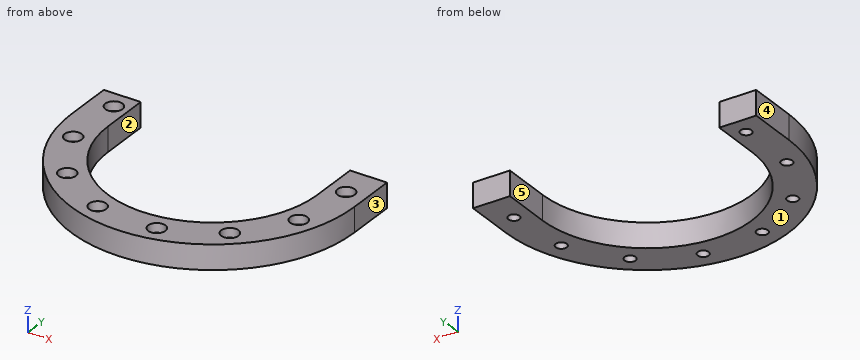
Autodesk Inventor part; units mm, degrees
ref_plane "YZ Plane" through (0, 0, 0) normal (1, 0, 0) x (0, 1, 0)
ref_plane "XZ Plane" through (0, 0, 0) normal (0, 1, 0) x (-1, 0, 0)
ref_plane "XY Plane" through (0, 0, 0) normal (0, 0, 1) x (1, 0, 0)
sketch "Sketch1" plane through (0, 0, 0) normal (0, 0, 1) x (1, 0, 0)
  circle A0 centre (0, 0) radius 200 construction
  line L0 (0, 200) -> (0, 230) construction
  line L1 (0, 200) -> (0, 170) construction
  circle A1 centre (0, 0) radius 170
  circle A2 centre (0, 0) radius 230
  line L2 (-170, 0) -> (-170, 80)
  line L3 (-170, 80) -> (-230, 80)
  line L4 (-230, 80) -> (-230, 0)
  line L5 (170, 0) -> (170, 80)
  line L6 (170, 80) -> (230, 80)
  line L7 (230, 80) -> (230, 0)
  dimension "d13" = 400
  dimension "d26" = 80
  dimension "d36" = 60
extrude "Extrusion1" add sketch "Sketch1" against normal blind 40 contours L5 L6 A2 L3 L2 A1 | L6 L7 A2 | A2 L4 L3 picked at (-188.7937, 40.2131)
sketch "Sketch4" plane through (0, 0, 0) normal (0, 0, 1) x (1, 0, 0)
  circle A0 centre (39.0181, -196.1571) radius 9
  line L0 (0, 0) -> (39.0181, -196.1571) construction
  line L1 (0, 0) -> (0, -276.8337) construction
  dimension "d17" = 18
  dimension "d27" = 200
  dimension "d35" = 11.25
extrude "Extrusion4" cut sketch "Sketch4" against normal through all
sketch "Sketch5" plane through (0, 0, 0) normal (0, 0, 1) x (1, 0, 0)
  circle A0 centre (39.0181, -196.1571) radius 9
  circle A1 centre (39.0181, -196.1571) radius 14
  point P0 (0, 0)
  dimension "d23" = 28
extrude "Extrusion5" cut sketch "Sketch5" against normal blind 15
pattern_circular "Circular Pattern3" count 8 over 202.5 about axis through (0, 0, 0) along (0, 0, -1) of "Extrusion4", "Extrusion5" both ways yes
equation "\"d13\" = Шпил_пласт_НОС_диам_центров"
equation "\"d27\" = 0.5 * Шпил_пласт_НОС_диам_центров"
properties part number "Постель 200"
Source: CAD feature listing. Evaluate the final solid. Frame: model axes, mm. Face numbers are marked on the shaded views. A direction names the side the tool comes from. Coordinates: 2 decimals unless noted, no trailing zeros. Loops run counter-clockwise (first coordinate to the right, second up) from the corner with the lowest first, then second, coordinate; pieces in that order, holes last. Notation, with made-up numbers: (82.5, -3) - (100.5, -3) arc R15 ccw to (100.5, 7) - close; hole circle Ø8 at (2, -38.75). An arc over 180 degrees is marked (long way). Return JSON: item names as keys, results as strings.
Q1. Contact query for flat-ended pins moving along their axis: P1, Ø14.5, axis at x = -193.66, y = -49.96, coming from the -Z side; P2, Ø12, axis at y = -189.5, z = -4, coming from the +X side; P3, Ø12, axis at y = -58.5, z = -27, coming from the +X side; P4, Ø14, axis at x = -191, y = 49, coming from the +Z side. Output: stop coordinate, or through.
Results:
{"P1": "through", "P2": "x = 138.66", "P3": "x = 223.93", "P4": "z = -15"}
Q2. Section C-C, the plane z = -26. Give the number of separate pieces and of enclosed holes in the cut face, plus the area to 3 significant figures.
Results:
{"separate pieces": "1", "enclosed holes": "8", "area": "45,300 mm2"}
Q3. Section A-A, the plane y = -25.5. Return loops of the section in (x, z).
Results:
{"outline": "(-228.58, -40) - (-168.08, -40) - (-168.08, 0) - (-228.58, 0) - close; (168.08, -40) - (228.58, -40) - (228.58, 0) - (168.08, 0) - close"}
Q4. Material intervals for line 1 along Y through (x, z) = (-205.5, -14); line 2 along Y through (x, z) = (-68.5, -10.5); line 3 along X through (y, z) = (-109.5, -27.5), sorted ascending.
Results:
{"line 1": "-103.29 to -57.43, -42.48 to 42.48, 57.43 to 80", "line 2": "-219.56 to -202.2, -178.91 to -155.59", "line 3": "-202.26 to -130.04, 130.04 to 202.26"}
Q5. Mould query, pull axis X, two halves, no side actions, for the marked faces 1, 2 and 3. Classes: released by +X, released by -X, zero draft, split by the parting line, or undercut.
Results:
{"face 1": "zero draft", "face 2": "undercut", "face 3": "released by +X"}
Q6. Access query for the marked faces 4 and 5. Directions: +Z, -Z, +X, -X, +Y, -Y. A direction counts if a zero-diameter tool reaches every point of the face in a straight line with its end or side. Return the directions, or none.
Results:
{"face 4": "+Z, -Z, -X, +Y, -Y", "face 5": "+Z, -Z, +Y"}
Q7. Section D-D, the plane x = 0. Return loops of the section in (y, z).
Results:
{"outline": "(-230, -40) - (-170, -40) - (-170, 0) - (-230, 0) - close"}
Q8. Section B-B, the plane y = 48. Return loops of the section in (x, z).
Results:
{"outline": "(-230, -40) - (-202.45, -40) - (-202.45, -15) - (-207.52, -15) - (-207.52, 0) - (-230, 0) - close; (-184.88, -40) - (-170, -40) - (-170, 0) - (-179.8, 0) - (-179.8, -15) - (-184.88, -15) - close; (170, -40) - (230, -40) - (230, 0) - (170, 0) - close"}
